from build123d import *

# Parameters (mm, degrees)
F0_W     = 373
F0_H     = 296
F1_DEPTH = 670
F2_T     = -10
F4_DEPTH = 25


with BuildPart() as f1:
    # F0 (on Front) → F1 (new body)
    with BuildSketch(Plane.XZ):
        Rectangle(F0_W, F0_H)
    extrude(amount=F1_DEPTH)

    # F2
    f2_openings = [f1.faces().sort_by_distance(p)[0] for p in [
        (0, 0, 0),
    ]]
    offset(amount=F2_T, openings=f2_openings)

    # F3 (on face) → F4 (cut)
    with BuildSketch(Plane.XZ.offset(670)):
        with BuildLine():
            ThreePointArc((-40, -125), (-45, -130), (-40, -135))
            Line((-40, -135), (40, -135))
            ThreePointArc((40, -135), (45, -130), (40, -125))
            Line((40, -125), (-40, -125))
        make_face()
    extrude(amount=-F4_DEPTH, mode=Mode.SUBTRACT)


solid = f1.part
Here's how the part is built. I have some questions about the finished solid (model axes, mm). A direction names the side the tool comes from. Give positions to 0.01 mm unless a question says otherwise; leave off trailing zeros. Loops run counter-clockwise (first coordinate to the right, second up) from the corner with the lowest first, then second, coordinate; pieces in that order, holes last. Notation, with made-up numbers: (63.5, 18) -> (68.5, 18) arc R34 cw to (68.5, 57) -> close; hole circle Ø3 at (87.5, 7.25). An arc over 180 degrees is marked (long way). Answer as a JSON object with one key per item and string values. Group by question number.
Item 1: Thinking about a two-plate mould opening in X: for faces 1 (the flat face through (-2, -325, 138)), 2 (the flat face through (186.5, -330, -2)), 3 (the flat face through (176.5, -325, -2)), 4 (the flat face through (-3, -670, 2)), which applies, pulls with the +X half, pulls with the -X half, needs draft (parallel to the pull), parting line crosses it, or undercut?
Item 2: On a 3-axis mill with a long thin cutter (end or side, diameter ignored), from which of +Z, -Z, +X, -X, +Y, -Y can I reach the whole of each face in a straight line? I mean faces 5 (the flat face through (-176.5, -325, -2)), 6 (the flat face through (-3, -330, 148)). Say none if no direction works.
Item 3: Imagine slicing it at A-A on x = 1.5. Write out the boundary of the cut face in (y, z).
Item 4: Will this pin go through, and if not, where does the flat tip stop? pin 1 (8 mm diameter, centred on x = 18.5, z = -52.5, fed in from +Y).
Item 5: Imagine slicing it at C-C on y = -157.5. Write out the boundary of the cut face in (x, z), then the cut area to 3 significant figures.
Item 6: I need wall thicknesses on L1, parallel to Z at x = -21, y = -56; L2, parallel to X at y = -209, z = -98; L3, parallel to Y at x = 91, z = 37.5. Which ranges of each line are inside material? Lowest first, please.
Item 7: Imagine slicing it at B-B on z = 63. Write out the boundary of the cut face in (x, y), then the cut area to 3 significant figures.
Item 8: Imagine slicing it at D-D on x = 138. Write out the boundary of the cut face in (y, z), then the cut area to 3 significant figures.
Answer list:
{
 "1": {"face 1": "undercut", "face 2": "pulls with the +X half", "face 3": "undercut", "face 4": "needs draft"},
 "2": {"face 5": "+Y", "face 6": "+Z, +X, -X, +Y, -Y"},
 "3": {"outline": "(-670, -148) -> (0, -148) -> (0, -138) -> (-660, -138) -> (-660, -135) -> (-670, -135) -> close; (-670, -125) -> (-660, -125) -> (-660, 138) -> (0, 138) -> (0, 148) -> (-670, 148) -> close"},
 "4": {"pin 1": "stops at y = -660"},
 "5": {"outline": "(-186.5, -148) -> (186.5, -148) -> (186.5, 148) -> (-186.5, 148) -> close; hole (-176.5, -138) -> (176.5, -138) -> (176.5, 138) -> (-176.5, 138) -> close", "area": "13,000 mm2"},
 "6": {"L1": "z = -148 to -138, 138 to 148", "L2": "x = -186.5 to -176.5, 176.5 to 186.5", "L3": "y = -670 to -660"},
 "7": {"outline": "(-186.5, -670) -> (186.5, -670) -> (186.5, 0) -> (176.5, 0) -> (176.5, -660) -> (-176.5, -660) -> (-176.5, 0) -> (-186.5, 0) -> close", "area": "16,900 mm2"},
 "8": {"outline": "(-670, -148) -> (0, -148) -> (0, -138) -> (-660, -138) -> (-660, 138) -> (0, 138) -> (0, 148) -> (-670, 148) -> close", "area": "16,200 mm2"}
}
